Here's the drawing with two shaded views (mm, measured from the low corner). I have some questions. Give positions to 0.01 mm unless a question says otherwise; leave off trailing zeros. Order: outer loops, then holes, each group sorted by start corner. A loop starts at its lowest first (then second) coordinate and runs counter-clockwise, first axis right, second up. Notation, with made-up numbers: (-8.75, 16.5) - (35.25, 16.5) arc R13 ccw to (35.25, 21.5) - close; hole circle Ø11 at (1, 63.25). An arc over 180 degrees is marked (long way). Use one line per item in the form item = value. Start each with the question number.
1) Suppose I cut it at C-C, the plane x = 1.75. Write out the boundary of the cut face in (y, z).
2) Suppose I cut it at B-B, the plane z = 2.75. Write out the boundary of the cut face in (x, y), and give its area (3 significant figures).
3) Please list where these lines run through material, in increasing order: probe 1 along X at (y, z) = (2.5, 3.35) (1 decimal); probe 2 along Y at (x, z) = (4.25, 0.4) (1 decimal); probe 3 along Y at (x, z) = (3.25, 1) (1 decimal).
4) For pin 1 (4.5 mm diameter, centred on x = 4, y = 4.62, fed in from +Z), with a flat end and sliding along its axis, tell me the tip position at first contact or that it passes through.
5) We'd pull the mould along X, two halves only. Please class the marked faces 1, 2, 3 and 4: released by +X, released by -X, zero draft, split by the parting line, or undercut.
6) Suppose I cut it at A-A, the plane y = 4.5. Write out the boundary of the cut face in (x, z).
7) Suppose I cut it at D-D, the plane x = 7.75. Write out the boundary of the cut face in (y, z) (1 decimal), and give its area (3 significant figures).
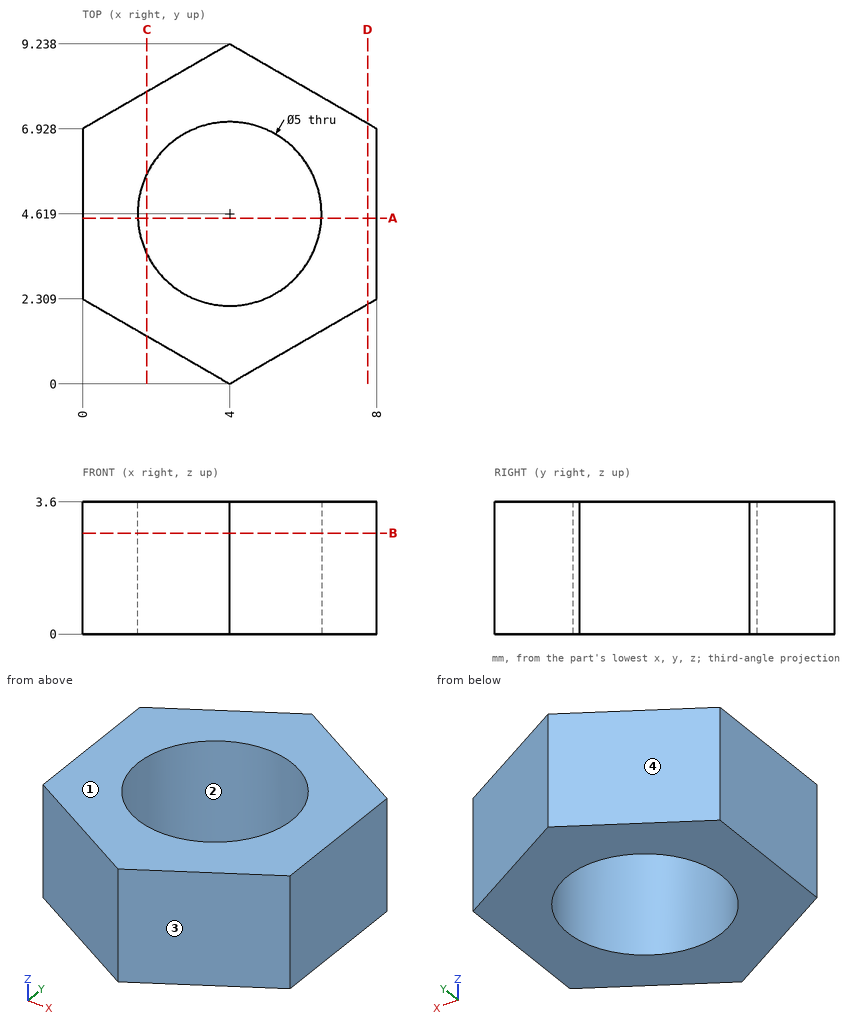
Result sheet:
q1.outline = (1.3, 0) - (3.53, 0) - (3.53, 3.6) - (1.3, 3.6) - close; (5.71, 0) - (7.94, 0) - (7.94, 3.6) - (5.71, 3.6) - close
q2.outline = (0, 2.31) - (4, 0) - (8, 2.31) - (8, 6.93) - (4, 9.24) - (0, 6.93) - close; hole circle Ø5 at (4, 4.62)
q2.area = 35.8 mm²
q3.probe_1 = 0 to 2.7, 5.3 to 8
q3.probe_2 = 0.1 to 2.1, 7.1 to 9.1
q3.probe_3 = 0.4 to 2.2, 7 to 8.8
q4.pin_1 = through
q5.face_1 = zero draft
q5.face_2 = undercut
q5.face_3 = released by +X
q5.face_4 = released by -X
q6.outline = (0, 0) - (1.5, 0) - (1.5, 3.6) - (0, 3.6) - close; (6.5, 0) - (8, 0) - (8, 3.6) - (6.5, 3.6) - close
q7.outline = (2.2, 0) - (7.1, 0) - (7.1, 3.6) - (2.2, 3.6) - close
q7.area = 17.7 mm²
